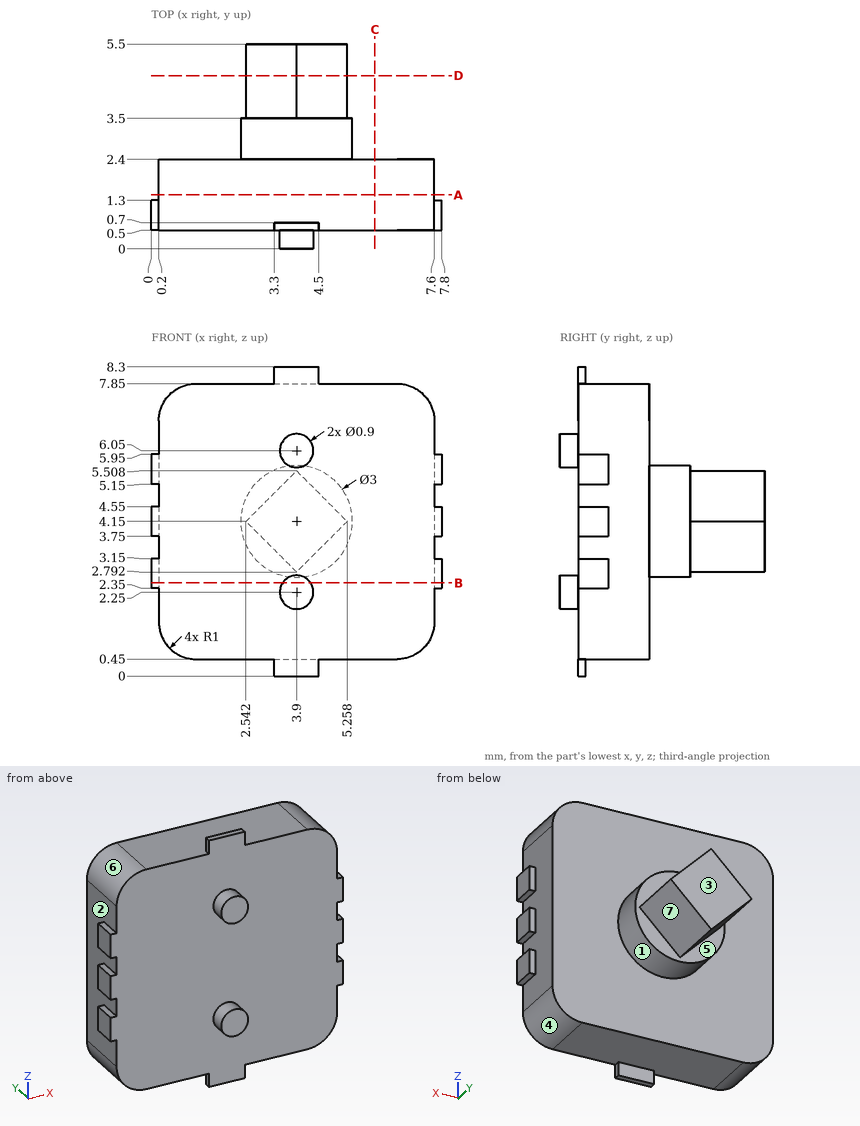
The figure shows three views and two pictorial views of one solid part (mm, origin at its lowest corner). Answer the questions. A direction names the side the tool comes from. Coordinates: 2 decimals unless noted, no trailing zeros. Loops run counter-clockwise (first coordinate to the right, second up) from the corner with the lowest first, then second, coordinate; pieces in that order, holes last. Notation, with made-up numbers: (89.5, 48) - (111.5, 48) arc R25 ccw to (111.5, 73) - close; hole circle Ø9 at (0, 9). An arc over 180 degrees is marked (long way). Use a Markdown table: item, result. Add a question column.
1) The mould has two halves that part along Z. Classify the marked faces 1, 2, 3 and 4: released by +Z, released by -Z, zero draft, split by the parting line, or undercut.
2) Given pin 1 (1.5 mm diameter, centred on x = 3.5, y = 1.5, fed in from -Z); pin 2 (2 mm diameter, centred on x = 1.5, y = 5, fed in from +Z); pin 3 (2.5 mm diameter, centred on x = 3.5, z = 3.5, fed in from -Y), each flat-ended and moving along its own axis, determine where each tip first touches the part or whether it passes through.
3) For the marked faces 5, 6 and 7, determine the directions among +Z, -Z, +X, -X, +Y, -Y from which every point of the face is accessible in a straight line to the end or side of a thin tool.
4) The part is cut by section A-A, the plane y = 1.45. Give the vertices of the cut face in (x, z).
5) The part is cut by section C-C, the plane x = 6. Give the vertices of the cut face in (y, z).
6) The part is cut by section D-D, the plane y = 4.65. Give the vertices of the cut face in (x, z).
7) Find the intervals of material crossed by line 1 (Z direction, x = 2.25, y = 1); line 2 (Y direction, x = 0.5, z = 6.5); line 3 (Y direction, x = 3.5, z = 3.5), in increasing order.
8) The part is cut by section B-B, the plane z = 2.5. Give the vertices of the cut face in (x, y).
Here are the results:
| question | item | result |
|---|---|---|
| 1 | face 1 | split by the parting line |
| 1 | face 2 | undercut |
| 1 | face 3 | zero draft |
| 1 | face 4 | released by -Z |
| 2 | pin 1 | stops at z = 0.45 |
| 2 | pin 2 | passes through |
| 2 | pin 3 | stops at y = 0 |
| 3 | face 5 | +Y |
| 3 | face 6 | +Z, -X, +Y, -Y |
| 3 | face 7 | -Z, +X, +Y |
| 4 | outline | (0.2, 1.45) arc R1 ccw to (1.2, 0.45) - (6.6, 0.45) arc R1 ccw to (7.6, 1.45) - (7.6, 6.85) arc R1 ccw to (6.6, 7.85) - (1.2, 7.85) arc R1 ccw to (0.2, 6.85) - close |
| 5 | outline | (0.5, 0.45) - (2.4, 0.45) - (2.4, 7.85) - (0.5, 7.85) - close |
| 6 | outline | (2.54, 4.15) - (3.9, 2.79) - (5.26, 4.15) - (3.9, 5.51) - close |
| 7 | line 1 | z = 0.45 to 7.85 |
| 7 | line 2 | y = 0.5 to 2.4 |
| 7 | line 3 | y = 0.5 to 5.5 |
| 8 | outline | (0, 0.5) - (3.53, 0.5) - (3.53, 0) - (4.27, 0) - (4.27, 0.5) - (7.8, 0.5) - (7.8, 1.3) - (7.6, 1.3) - (7.6, 2.4) - (0.2, 2.4) - (0.2, 1.3) - (0, 1.3) - close |
